Check sheet for the modelled part. Datum: model origin and axes. Units: mm. Round coordinates to 2 decimals unless told otherwise and drop trailing zeros. Write each loop counter-clockwise with the first axis right and the second up, starting at its lowest first coordinate (ties: lowest second). Pieces come first, ordered by that corner, then holes. Notation, with made-up numbers: (3.25, 35) -> (24.25, 35) arc R32 ccw to (24.25, 61) -> close; hole circle Ø1 at (83.5, 3). An arc over 180 degrees is marked (long way). One line per item, written item: value.
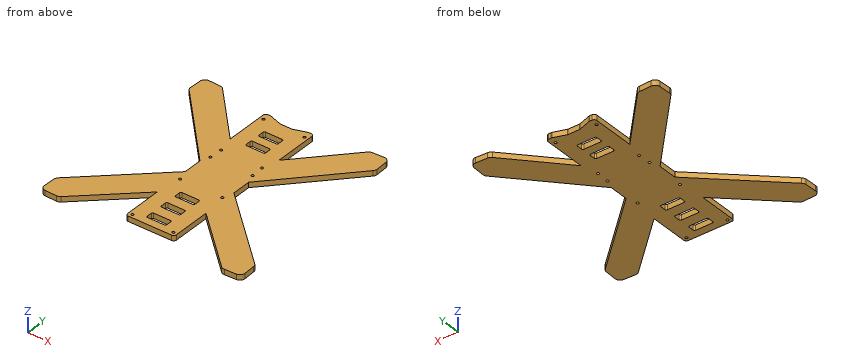
from build123d import *

# Parameters (mm, degrees)
F0_R     = 1
F1_DEPTH = 4


with BuildPart() as f1:
    # F0 (on Top) → F1 (new body)
    with BuildSketch(Plane.XY):
        with BuildLine():
            ThreePointArc((-16.7198, 64.620168), (-18.134014, 64.034382), (-18.7198, 62.620168))
            Line((-18.7198, 62.620168), (-18.7198, 29.936337))
            Line((-18.7198, 29.936337), (-55.794644, 70.026107))
            ThreePointArc((-55.794644, 70.026107), (-56.99751, 70.899639), (-58.443099, 71.246361))
            Line((-58.443099, 71.246361), (-67.416509, 71.596964))
            ThreePointArc((-67.416509, 71.596964), (-70.152099, 70.587073), (-71.372352, 67.938617))
            Line((-71.372352, 67.938617), (-71.722956, 58.965208))
            ThreePointArc((-71.722956, 58.965208), (-71.490081, 57.496973), (-70.713064, 56.229618))
            Line((-70.713064, 56.229618), (-18.7198, 0.008261))
            Line((-18.7198, 0.008261), (-18.7198, -14.626099))
            Line((-18.7198, -14.626099), (-75.507393, -67.143016))
            ThreePointArc((-75.507393, -67.143016), (-76.380925, -68.345882), (-76.727646, -69.791472))
            Line((-76.727646, -69.791472), (-77.078249, -78.764881))
            ThreePointArc((-77.078249, -78.764881), (-76.068358, -81.500471), (-73.419902, -82.720725))
            Line((-73.419902, -82.720725), (-64.446493, -83.071328))
            ThreePointArc((-64.446493, -83.071328), (-62.978258, -82.838454), (-61.710903, -82.061437))
            Line((-61.710903, -82.061437), (-18.7198, -42.303453))
            Line((-18.7198, -42.303453), (-18.7198, -71.62687))
            ThreePointArc((-18.7198, -71.62687), (-18.134014, -73.041084), (-16.7198, -73.62687))
            Line((-16.7198, -73.62687), (0, -73.62687))
            Line((0, -73.62687), (16.7198, -73.62687))
            ThreePointArc((16.7198, -73.62687), (18.134014, -73.041084), (18.7198, -71.62687))
            Line((18.7198, -71.62687), (18.7198, -42.303453))
            Line((18.7198, -42.303453), (61.710903, -82.061437))
            ThreePointArc((61.710903, -82.061437), (62.978258, -82.838454), (64.446493, -83.071328))
            Line((64.446493, -83.071328), (73.419902, -82.720725))
            ThreePointArc((73.419902, -82.720725), (76.068358, -81.500471), (77.078249, -78.764881))
            Line((77.078249, -78.764881), (76.727646, -69.791472))
            ThreePointArc((76.727646, -69.791472), (76.380925, -68.345882), (75.507393, -67.143016))
            Line((75.507393, -67.143016), (18.7198, -14.626099))
            Line((18.7198, -14.626099), (18.7198, 0.008261))
            Line((18.7198, 0.008261), (70.713064, 56.229618))
            ThreePointArc((70.713064, 56.229618), (71.490081, 57.496973), (71.722956, 58.965208))
            Line((71.722956, 58.965208), (71.372352, 67.938617))
            ThreePointArc((71.372352, 67.938617), (70.152099, 70.587073), (67.416509, 71.596964))
            Line((67.416509, 71.596964), (58.443099, 71.246361))
            ThreePointArc((58.443099, 71.246361), (56.99751, 70.899639), (55.794644, 70.026107))
            Line((55.794644, 70.026107), (18.7198, 29.936337))
            Line((18.7198, 29.936337), (18.7198, 62.620168))
            ThreePointArc((18.7198, 62.620168), (18.134014, 64.034382), (16.7198, 64.620168))
            Line((16.7198, 64.620168), (14.7254, 64.620168))
            ThreePointArc((14.7254, 64.620168), (14.399241, 64.593394), (14.081814, 64.513788))
            Line((14.081814, 64.513788), (4.877257, 61.385427))
            ThreePointArc((4.877257, 61.385427), (4.55983, 61.305821), (4.23367, 61.279047))
            Line((4.23367, 61.279047), (0, 61.279047))
            Line((0, 61.279047), (-4.23367, 61.279047))
            ThreePointArc((-4.23367, 61.279047), (-4.55983, 61.305821), (-4.877257, 61.385427))
            Line((-4.877257, 61.385427), (-14.081814, 64.513788))
            ThreePointArc((-14.081814, 64.513788), (-14.399241, 64.593394), (-14.7254, 64.620168))
            Line((-14.7254, 64.620168), (-16.7198, 64.620168))
        make_face()
        with Locations((-15.7198, -70.62687)):
            Circle(F0_R, mode=Mode.SUBTRACT)
        with Locations((-16.2198, -22.879832)):
            Circle(F0_R, mode=Mode.SUBTRACT)
        with BuildLine():
            Line((6.5, -67.62687), (0, -67.62687))
            Line((0, -67.62687), (-6.5, -67.62687))
            ThreePointArc((-6.5, -67.62687), (-7.207107, -67.333977), (-7.5, -66.62687))
            Line((-7.5, -66.62687), (-7.5, -62.63247))
            ThreePointArc((-7.5, -62.63247), (-7.207107, -61.925364), (-6.5, -61.63247))
            Line((-6.5, -61.63247), (0, -61.63247))
            Line((0, -61.63247), (6.5, -61.63247))
            ThreePointArc((6.5, -61.63247), (7.207107, -61.925364), (7.5, -62.63247))
            Line((7.5, -62.63247), (7.5, -66.62687))
            ThreePointArc((7.5, -66.62687), (7.207107, -67.333977), (6.5, -67.62687))
        make_face(mode=Mode.SUBTRACT)
        with Locations((15.7198, -70.62687)):
            Circle(F0_R, mode=Mode.SUBTRACT)
        with BuildLine():
            Line((6.493, -53.61877), (0, -53.61877))
            Line((0, -53.61877), (-6.493, -53.61877))
            ThreePointArc((-6.493, -53.61877), (-7.200107, -53.325877), (-7.493, -52.61877))
            Line((-7.493, -52.61877), (-7.493, -48.62437))
            ThreePointArc((-7.493, -48.62437), (-7.200107, -47.917264), (-6.493, -47.62437))
            Line((-6.493, -47.62437), (0, -47.62437))
            Line((0, -47.62437), (6.493, -47.62437))
            ThreePointArc((6.493, -47.62437), (7.200107, -47.917264), (7.493, -48.62437))
            Line((7.493, -48.62437), (7.493, -52.61877))
            ThreePointArc((7.493, -52.61877), (7.200107, -53.325877), (6.493, -53.61877))
        make_face(mode=Mode.SUBTRACT)
        with BuildLine():
            Line((6.493, -39.62687), (0, -39.62687))
            Line((0, -39.62687), (-6.493, -39.62687))
            ThreePointArc((-6.493, -39.62687), (-7.200107, -39.333977), (-7.493, -38.62687))
            Line((-7.493, -38.62687), (-7.493, -34.63247))
            ThreePointArc((-7.493, -34.63247), (-7.200107, -33.925364), (-6.493, -33.63247))
            Line((-6.493, -33.63247), (0, -33.63247))
            Line((0, -33.63247), (6.493, -33.63247))
            ThreePointArc((6.493, -33.63247), (7.200107, -33.925364), (7.493, -34.63247))
            Line((7.493, -34.63247), (7.493, -38.62687))
            ThreePointArc((7.493, -38.62687), (7.200107, -39.333977), (6.493, -39.62687))
        make_face(mode=Mode.SUBTRACT)
        with Locations((16.2198, -22.879832)):
            Circle(F0_R, mode=Mode.SUBTRACT)
        with Locations((-16.2198, 7.120168)):
            Circle(F0_R, mode=Mode.SUBTRACT)
        with Locations((-15.7226, 16.995168)):
            Circle(F0_R, mode=Mode.SUBTRACT)
        with Locations((-15.7226, 59.057568)):
            Circle(F0_R, mode=Mode.SUBTRACT)
        with Locations((16.2198, 7.120168)):
            Circle(F0_R, mode=Mode.SUBTRACT)
        with Locations((15.7226, 16.995168)):
            Circle(F0_R, mode=Mode.SUBTRACT)
        with BuildLine():
            Line((-6.5, 36.279047), (0, 36.279047))
            Line((0, 36.279047), (6.5, 36.279047))
            ThreePointArc((6.5, 36.279047), (7.207107, 35.986154), (7.5, 35.279047))
            Line((7.5, 35.279047), (7.5, 31.279047))
            ThreePointArc((7.5, 31.279047), (7.207107, 30.57194), (6.5, 30.279047))
            Line((6.5, 30.279047), (0, 30.279047))
            Line((0, 30.279047), (-6.5, 30.279047))
            ThreePointArc((-6.5, 30.279047), (-7.207107, 30.57194), (-7.5, 31.279047))
            Line((-7.5, 31.279047), (-7.5, 35.279047))
            ThreePointArc((-7.5, 35.279047), (-7.207107, 35.986154), (-6.5, 36.279047))
        make_face(mode=Mode.SUBTRACT)
        with BuildLine():
            Line((6.5, 42.914193), (-6.5, 42.914193))
            ThreePointArc((-6.5, 42.914193), (-7.207107, 43.207086), (-7.5, 43.914193))
            Line((-7.5, 43.914193), (-7.5, 47.908593))
            ThreePointArc((-7.5, 47.908593), (-7.207107, 48.6157), (-6.5, 48.908593))
            Line((-6.5, 48.908593), (6.5, 48.908593))
            ThreePointArc((6.5, 48.908593), (7.207107, 48.6157), (7.5, 47.908593))
            Line((7.5, 47.908593), (7.5, 43.914193))
            ThreePointArc((7.5, 43.914193), (7.207107, 43.207086), (6.5, 42.914193))
        make_face(mode=Mode.SUBTRACT)
        with Locations((15.7226, 59.057568)):
            Circle(F0_R, mode=Mode.SUBTRACT)
    extrude(amount=F1_DEPTH)


solid = f1.part
Item 1: Sectioned sample at C-C on y = 25. Enter the section's corners in (x, z), and give its area (3 significant figures).
Answer:
outline: (-41.83, 0) -> (41.83, 0) -> (41.83, 4) -> (-41.83, 4) -> close
area: 335 mm^2
Item 2: Sectioned sample at A-A on x = 25. Enter the section's corners in (y, z), and give its area (3 significant figures).
Answer:
outline: (-48.11, 0) -> (-20.43, 0) -> (-20.43, 4) -> (-48.11, 4) -> close; (6.8, 0) -> (36.73, 0) -> (36.73, 4) -> (6.8, 4) -> close
area: 230 mm^2
Item 3: Depth check by flat-ended pin: P1, Ø1.2, axis at y = 39, z = 1.5, coming from the -X side; P2, Ø1.2, axis at x = 3, z = 1.5, coming from the -Y side; P3, Ø10, axis at x = -56, y = -36, coming from the -Z side; P4, Ø1.2, axis at y = -54.5, z = 3, coming from the -X side. Enter the tip coordinate at first touch or a pass-through.
Answer:
P1: stops at x = -55.33
P2: stops at y = -73.63
P3: passes through
P4: stops at x = -62.49
Item 4: Sectioned sample at B-B on z = 2.85. Count the separate pieces of the cut face and the enclosed holes in it, and give its area (3 significant figures).
Answer:
separate pieces: 1
enclosed holes: 15
area: 10,600 mm^2
Item 5: Thickness scan on line 1 (X direction, y = -44.5, z = 2.4); line 2 (X direction, y = 17.5, z = 3.2); line 3 (X direction, y = 30.5, z = 3). Record the ranges inside material, lowest first.
Answer:
line 1: x = -51.02 to -21.09, -18.72 to 18.72, 21.09 to 51.02
line 2: x = -34.9 to -16.59, -14.86 to 14.86, 16.59 to 34.9
line 3: x = -46.92 to -19.24, -18.72 to -7.13, 7.13 to 18.72, 19.24 to 46.92
